Design review of the part built by this model. Coordinates are the model's own, in mm. A direction names the side the tool comes from. Coordinates: 2 decimals unless noted, no trailing zeros. Loops run counter-clockwise (first coordinate to the right, second up) from the corner with the lowest first, then second, coordinate; pieces in that order, holes last. Notation, with made-up numbers: (41, 34.5) -> (71, 34.5) arc R18 cw to (71, 55.5) -> close; hole circle Ø7 at (19.5, 36). An arc over 180 degrees is marked (long way). Use one line per item in the form item = value. Start each with the question number.
1. Consider section A-A (y = 0). State the section outline as (x, z) points, then the cut area to 3 significant figures.
2. Machinability: for faces 1 (the face through (-3, 0, 11)), 2 (the face through (1, 3, -10)), 3 (the face through (-2, 2, -12)), which of the approach directions +Z, -Z, +X, -X, +Y, -Y give a long, thin tool a straight path to every point of the face, cutting with its end or side? Answer none if there is none.
3. Wall thickness on line 1 (Y direction, x = 0, z = -3.5); line 2 (X direction, y = -0.5, z = 6.5); line 3 (Y direction, x = 1.75, z = 1.75): over which ranges is each line inside the solid? List them lowest first. Write a range as from..to.
4. For pin 1 (1.5 mm diameter, centred on x = -2, z = -3.5, fed in from -Y); pin 2 (4 mm diameter, centred on x = -3, z = -3.5, fed in from -Y); pin 3 (1.5 mm diameter, centred on y = -1.5, z = -4, fed in from +X), all flat-tipped, find the tip position at first contact; note any pin that passes through.
5. Consider section C-C (z = -4). State the section outline as (x, y) points.
6. Consider section D-D (y = 2.5). State the section outline as (x, z) points.
from build123d import *

# Parameters (mm, degrees)
SKETCH1_R           = 4
BOSS_EXTRUDE1_DEPTH = 10
SKETCH2_R           = 3
BOSS_EXTRUDE2_DEPTH = 2
SKETCH3_R           = 2
CUT_EXTRUDE1_DEPTH  = 25
CHAMFER1_SIZE       = 0.2


with BuildPart() as part:
    # Sketch1 → Boss-Extrude1 (new body)
    with BuildSketch(Plane.XY):
        Circle(SKETCH1_R)
    boss_extrude1 = extrude(amount=BOSS_EXTRUDE1_DEPTH)

    # Sketch2 → Boss-Extrude2 (add)
    with BuildSketch(Plane.XY.offset(10)):
        Circle(SKETCH2_R)
    boss_extrude2 = extrude(amount=BOSS_EXTRUDE2_DEPTH)

    # Mirror1: Boss-Extrude1, Boss-Extrude2 across plane
    add(boss_extrude1.mirror(Plane.XY))
    add(boss_extrude2.mirror(Plane.XY))

    # Sketch3 → Cut-Extrude1 (cut, through all)
    with BuildSketch(Plane.XY.offset(12)):
        Circle(SKETCH3_R)
    extrude(amount=-CUT_EXTRUDE1_DEPTH, mode=Mode.SUBTRACT)

    # Chamfer1
    chamfer1_edges = [part.edges().sort_by_distance(p)[0] for p in [
        (-2, 0, -12),
        (-2, 0, 12),
    ]]
    chamfer(chamfer1_edges, length=CHAMFER1_SIZE)


solid = part.part
Geometry check:
q1.outline = (-4, -10) -> (-3, -10) -> (-3, -12) -> (-2.2, -12) -> (-2, -11.8) -> (-2, 11.8) -> (-2.2, 12) -> (-3, 12) -> (-3, 10) -> (-4, 10) -> close; (2, -11.8) -> (2.2, -12) -> (3, -12) -> (3, -10) -> (4, -10) -> (4, 10) -> (3, 10) -> (3, 12) -> (2.2, 12) -> (2, 11.8) -> close
q1.area = 87.9 mm²
q2.face_1 = +Z
q2.face_2 = -Z
q2.face_3 = -Z, +X, -X, +Y, -Y
q3.line_1 = -4..-2, 2..4
q3.line_2 = -3.97..-1.94, 1.94..3.97
q3.line_3 = -3.6..-0.97, 0.97..3.6
q4.pin_1 = -3.8
q4.pin_2 = -3.87
q4.pin_3 = 3.93
q5.outline = circle Ø8 at (0, 0); hole circle Ø4 at (0, 0)
q6.outline = (-3.12, -10) -> (-1.66, -10) -> (-1.66, -12) -> (1.66, -12) -> (1.66, -10) -> (3.12, -10) -> (3.12, 10) -> (1.66, 10) -> (1.66, 12) -> (-1.66, 12) -> (-1.66, 10) -> (-3.12, 10) -> close
